The drawing under review shows one solid part. Ordinate dimensions are in mm from its lowest x, y, z. A direction names the side the tool comes from. Give positions to 0.01 mm unless a question says otherwise; leave off trailing zeros. Write each loop counter-clockwise with the first axis right and the second up, starting at its lowest first coordinate (ties: lowest second). Pieces come first, ordered by that corner, then holes. Notation, with made-up numbers: (23, 30) -> (60, 30) arc R17 cw to (60, 54) -> close; hole circle Ø6 at (-14, 84). An arc over 180 degrees is marked (long way). Use CSV: the item, a comma, the result in double quotes.
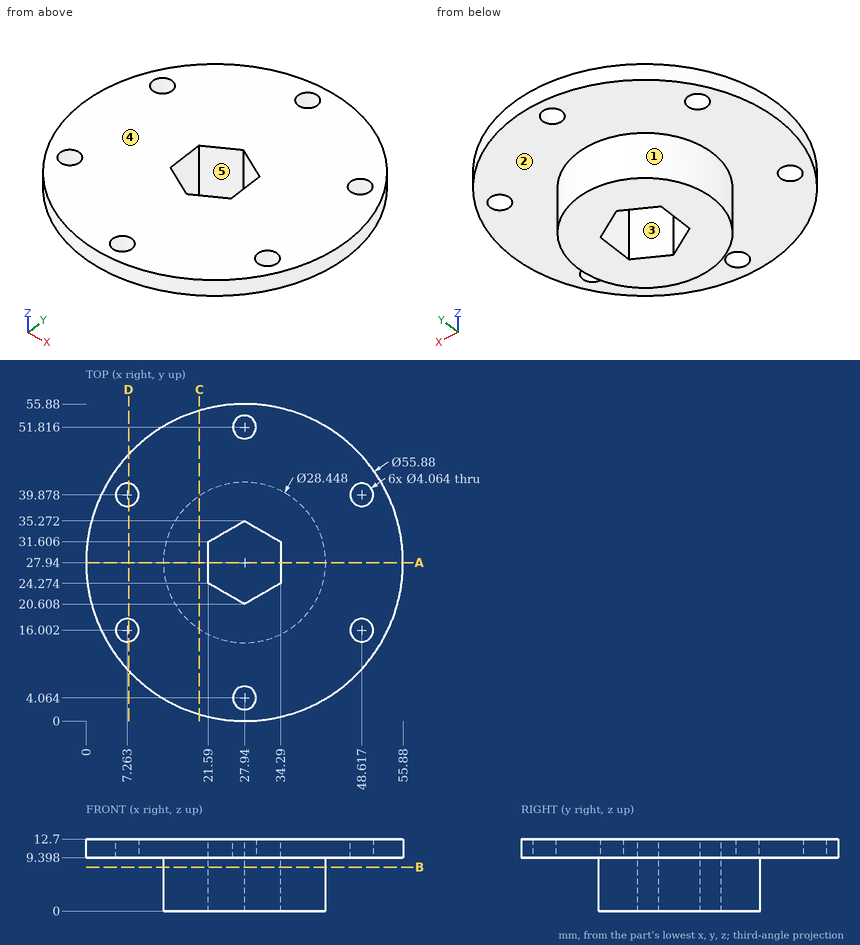
(1) Take a section at C-C (x = 20). Write out the cut boundary in (y, z), then the cut area to 3 significant figures.
Established:
outline,"(1.15, 9.4) -> (16.14, 9.4) -> (16.14, 0) -> (39.74, 0) -> (39.74, 9.4) -> (54.73, 9.4) -> (54.73, 12.7) -> (1.15, 12.7) -> close"
area,"399 mm2"
(2) Take a section at B-B (z = 7.75). Write out the cut boundary in (x, y).
Established:
outline,"circle Ø28.45 at (27.94, 27.94); hole (21.59, 24.27) -> (27.94, 20.61) -> (34.29, 24.27) -> (34.29, 31.61) -> (27.94, 35.27) -> (21.59, 31.61) -> close"
(3) Take a section at A-A (y = 27.94). Write out the cut boundary in (x, z).
Established:
outline,"(0, 9.4) -> (13.72, 9.4) -> (13.72, 0) -> (21.59, 0) -> (21.59, 12.7) -> (0, 12.7) -> close; (34.29, 0) -> (42.16, 0) -> (42.16, 9.4) -> (55.88, 9.4) -> (55.88, 12.7) -> (34.29, 12.7) -> close"
(4) Take a section at D-D (x = 7.5). Write out the cut boundary in (y, z).
Established:
outline,"(8.89, 9.4) -> (13.98, 9.4) -> (13.98, 12.7) -> (8.89, 12.7) -> close; (18.02, 9.4) -> (37.86, 9.4) -> (37.86, 12.7) -> (18.02, 12.7) -> close; (41.9, 9.4) -> (46.99, 9.4) -> (46.99, 12.7) -> (41.9, 12.7) -> close"
(5) Clearance check with flat-ended pins moving along their axes: pin 1 (2 mm diameter, centred on x = 14, z = 5.5, fed in from +Y) (1 decimal); pin 2 (6 mm diameter, centred on x = 24, z = 9, fed in from +Y); pin 3 (5.5 mm diameter, centred on x = 7.26, y = 16, fed in from -Z); pin 4 (5.5 mm diameter, centred on x = 27.94, y = 51.816, fed in from +Z). State where each tip first meets the part, or that it passes through.
Established:
pin 1,"stops at y = 33.8"
pin 2,"stops at y = 55.86"
pin 3,"stops at z = 9.4"
pin 4,"stops at z = 12.7"
(6) For line 1 along Z through (x, y) = (16.5, 44.5); line 2 along X through (y, z) = (32, 10.75) (1 decimal); line 3 along Y through (x, z) = (31, 12.25) (1 decimal), list the stretches that pass through material, from the lowest coordinate up. Write a range as [from, to].
Established:
line 1,"z = [9.4, 12.7]"
line 2,"x = [0.3, 22.3], [33.6, 55.6]"
line 3,"y = [0.2, 22.4], [33.5, 55.7]"
(7) Mouldability with a two-part tool opening along Y and no side actions: class the marked faces 1, 2 and 3 as +Y half, -Y half, draft (parallel to the pull), parting line (faces both ways), or undercut.
Established:
face 1,"parting line"
face 2,"draft"
face 3,"undercut"
(8) Tool access review of the marked faces 4 and 5: name each direction out of +Z, -Z, +X, -X, +Y, -Y from which nothing blocks a thin tool from reaching the whole face with its end or side.
Established:
face 4,"+Z, +X, -X, +Y, -Y"
face 5,"+Z, -Z"
